from build123d import *

# Parameters (mm, degrees)
EXTRUDE_1_DEPTH              = 72
HOLE_WIZARD_M3_1_D           = 3.6
HOLE_WIZARD_M3_1_DEPTH       = 4
HOLE_WIZARD_M3_1_CBORE_D     = 7
HOLE_WIZARD_M3_1_CBORE_DEPTH = 2


with BuildPart() as part:
    # 草图1 → 凸台-拉伸1 (new body)
    with BuildSketch(Plane(origin=(0, 72, 0), x_dir=(1, 0, 0), z_dir=(0, 1, 0))):
        with BuildLine():
            Line((1135, -1.494230428), (1135, 2.25))
            Line((1135, 2.25), (1125, 2.25))
            Line((1125, 2.25), (1125, -1.494230428))
            ThreePointArc((1125, -1.494230428), (1130, -1.75), (1135, -1.494230428))
        make_face()
    extrude(amount=-EXTRUDE_1_DEPTH)

    # M3 六角头机械螺钉的柱形沉头孔1
    with Locations(Plane(origin=(1130, 60, 1.75), x_dir=(1, 0, 0), z_dir=(0, 0, 1))):
        with Locations((0, 0)):
            CounterBoreHole(HOLE_WIZARD_M3_1_D / 2, HOLE_WIZARD_M3_1_CBORE_D / 2, HOLE_WIZARD_M3_1_CBORE_DEPTH, depth=HOLE_WIZARD_M3_1_DEPTH)


solid = part.part
Read the model definition and answer for the solid it produces. Units are mm, in the model's axes. A direction names the side the tool comes from. Round coordinates to 2 decimals unless told otherwise and drop trailing zeros. Write each loop counter-clockwise with the first axis right and the second up, starting at its lowest first coordinate (ties: lowest second). Pieces come first, ordered by that corner, then holes. Notation, with made-up numbers: (-15.75, 56) - (36.25, 56) arc R27 cw to (36.25, 82) - close; hole circle Ø8 at (-11.5, -38). An arc over 180 degrees is marked (long way). Use a Markdown table: item, result.
(1) Straight lines are drawn through the part: line 1 along X through (y, z) = (60, 0.3); line 2 along Y through (x, z) = (1130, 0.75); line 3 along Y through (x, z) = (1130, -1.8). For each, find the intervals that lie inside material, in ascending order. Write a range as [from, to].
Reported:
| item | result |
|---|---|
| line 1 | [1125, 1126.5], [1133.5, 1135] |
| line 2 | [0, 56.5], [63.5, 72] |
| line 3 | [0, 58.2], [61.8, 72] |
(2) The part is cut by section C-C (y = 50). Write down the section's boundary in (x, z), then the cut area to 3 significant figures.
Reported:
| item | result |
|---|---|
| outline | (1125, -2.25) - (1135, -2.25) - (1135, 1.49) arc R49 ccw to (1125, 1.49) - close |
| area | 39.1 mm2 |
(3) The mould has two halves that part along X. Classify faces 3 (the flat face through (1129, 62, -0.25)), 4 (the flat face through (1130, 37, -2.25)), 5 (the flat face through (1125, 37, 0)): released by +X, released by -X, zero draft, split by the parting line, or undercut.
Reported:
| item | result |
|---|---|
| face 3 | undercut |
| face 4 | zero draft |
| face 5 | released by -X |
(4) The part is cut by section A-A (x = 1130). Write down the section's boundary in (y, z).
Reported:
| item | result |
|---|---|
| outline | (0, -2.25) - (58.2, -2.25) - (58.2, -0.25) - (56.5, -0.25) - (56.5, 1.75) - (0, 1.75) - close; (61.8, -2.25) - (72, -2.25) - (72, 1.75) - (63.5, 1.75) - (63.5, -0.25) - (61.8, -0.25) - close |
(5) Which of the six approach directions +Z, -Z, +X, -X, +Y, -Y give full straight-line access (tool end or side, diameter ignored) to faces 1 (the flat face through (1135, 37, 0)), 2 (the cylindrical face through (1126.503, 60.154, 0.766))?
Reported:
| item | result |
|---|---|
| face 1 | +Z, -Z, +X, +Y, -Y |
| face 2 | +Z |
(6) The part is cut by section B-B (y = 60). Write down the section's boundary in (x, z).
Reported:
| item | result |
|---|---|
| outline | (1125, -2.25) - (1128.2, -2.25) - (1128.2, -0.25) - (1126.5, -0.25) - (1126.5, 1.62) arc R49 ccw to (1125, 1.49) - close; (1131.8, -2.25) - (1135, -2.25) - (1135, 1.49) arc R49 ccw to (1133.5, 1.62) - (1133.5, -0.25) - (1131.8, -0.25) - close |
(7) Each of these flat-tipped pins is pushed along its axis until it touches: pin 1 Ø2 at (x, z) = (1126.5, 0) entering from -Y; pin 2 Ø4 at (x, y) = (1130, 60) entering from +Z. Where does it stop, or does it pass through?
Reported:
| item | result |
|---|---|
| pin 1 | y = 0 |
| pin 2 | z = -0.25 |
